Verification items for the finished model (mm, model axes). A direction names the side the tool comes from. Coordinates: 2 decimals unless noted, no trailing zeros. Write each loop counter-clockwise with the first axis right and the second up, starting at its lowest first coordinate (ties: lowest second). Pieces come first, ordered by that corner, then holes. Notation, with made-up numbers: (83.25, 50) -> (120.25, 50) arc R18 cw to (120.25, 70) -> close; hole circle Ø11 at (19, -29). An arc over 180 degrees is marked (long way). Use CSV: the item, a comma, the result in double quotes.
```python
from build123d import *

# Parameters (mm, degrees)
F0_W     = 33
F0_H     = 80
F1_DEPTH = 70
F3_DEPTH = 60
F4_R     = 6.5
F4_R_2   = 4.5
F4_R_3   = 5.125
F5_DEPTH = 2.5


with BuildPart() as f1:
    # F0 (on Top) → F1 (new body)
    with BuildSketch(Plane.XY):
        with Locations((-71, -15)):
            Rectangle(F0_W, F0_H)
    extrude(amount=F1_DEPTH)

    # F2 (on face) → F3 (cut)
    with BuildSketch(Plane.XY.offset(70)):
        Polygon((-72.875, 20), (-72.875, 15), (-83, 15), (-83, -22), (-77, -22), (-77, -50), (-71, -50), (-65, -50), (-65, -22), (-59, -22), (-59, 15), (-69.125, 15), (-69.125, 20), (-71, 20), align=None)
    extrude(amount=-F3_DEPTH, mode=Mode.SUBTRACT)

    # F4 (on face) → F5 (cut)
    with BuildSketch(Plane.XY.offset(10)):
        with Locations((-71, 4.75)):
            Circle(F4_R)
        with Locations((-71, 4.75)):
            Circle(F4_R_2, mode=Mode.SUBTRACT)
        with Locations((-71, -11.025)):
            Circle(F4_R_3)
    extrude(amount=-F5_DEPTH, mode=Mode.SUBTRACT)


solid = f1.part
```
1) Set-up check for faces 3 (the flat face through (-71, -14, 0)), 4 (the flat face through (-83, -3, 40)): record each of +Z, -Z, +X, -X, +Y, -Y from which the full face is reachable in a straight line by a thin tool's end or side.
Return value:
face 3,"-Z, +X, -X, +Y, -Y"
face 4,"+Z"
2) Gauge pin test, flat end, axial feed: pin 1 (8 mm diameter, centred on x = -71, y = 4.75, fed in from +Z). Record the tip position at first contact, or that the pin passes through.
Return value:
pin 1,"z = 10"
3) Cross-section at A-A (z = 26). Record the boundary of the cut face in (x, y) (3 decimals), plus the area to 3 significant figures.
Return value:
outline,"(-87.5, -55) -> (-54.5, -55) -> (-54.5, 25) -> (-87.5, 25) -> close; hole (-83, -22) -> (-77, -22) -> (-77, -50) -> (-65, -50) -> (-65, -22) -> (-59, -22) -> (-59, 15) -> (-69.125, 15) -> (-69.125, 20) -> (-72.875, 20) -> (-72.875, 15) -> (-83, 15) -> close"
area,"1,400 mm2"
4) Cross-section at D-D (y = 19). Record the boundary of the cut face in (x, z) (3 decimals).
Return value:
outline,"(-87.5, 0) -> (-54.5, 0) -> (-54.5, 70) -> (-69.125, 70) -> (-69.125, 10) -> (-72.875, 10) -> (-72.875, 70) -> (-87.5, 70) -> close"
5) Cross-section at B-B (y = -5). Record the boundary of the cut face in (x, z), plus the area to 3 significant figures.
Return value:
outline,"(-87.5, 0) -> (-54.5, 0) -> (-54.5, 70) -> (-59, 70) -> (-59, 10) -> (-83, 10) -> (-83, 70) -> (-87.5, 70) -> close"
area,"870 mm2"
6) Cross-section at C-C (x = -71). Record the boundary of the cut face in (y, z).
Return value:
outline,"(-55, 0) -> (25, 0) -> (25, 70) -> (20, 70) -> (20, 10) -> (11.25, 10) -> (11.25, 7.5) -> (9.25, 7.5) -> (9.25, 10) -> (0.25, 10) -> (0.25, 7.5) -> (-1.75, 7.5) -> (-1.75, 10) -> (-5.9, 10) -> (-5.9, 7.5) -> (-16.15, 7.5) -> (-16.15, 10) -> (-50, 10) -> (-50, 70) -> (-55, 70) -> close"
7) Mould release check, pull along X, two halves, no side actions. Record for faces 1 (the flat face through (-64, -23, 70)), 2 (the flat face through (-69.6, 9.2, 7.5)): released by +X, released by -X, zero draft, split by the parting line, or undercut.
Return value:
face 1,"zero draft"
face 2,"undercut"
8) Scan lines: L1, parallel to Y at x = -71, z = 9.55; L2, parallel to Y at x = -65.5, z = 30.5; L3, parallel to X at y = -4, z = 29. Record each from-to range of solid material in increasing order.
Return value:
L1,"-55 to -16.15, -5.9 to -1.75, 0.25 to 9.25, 11.25 to 25"
L2,"-55 to -50, 15 to 25"
L3,"-87.5 to -83, -59 to -54.5"
